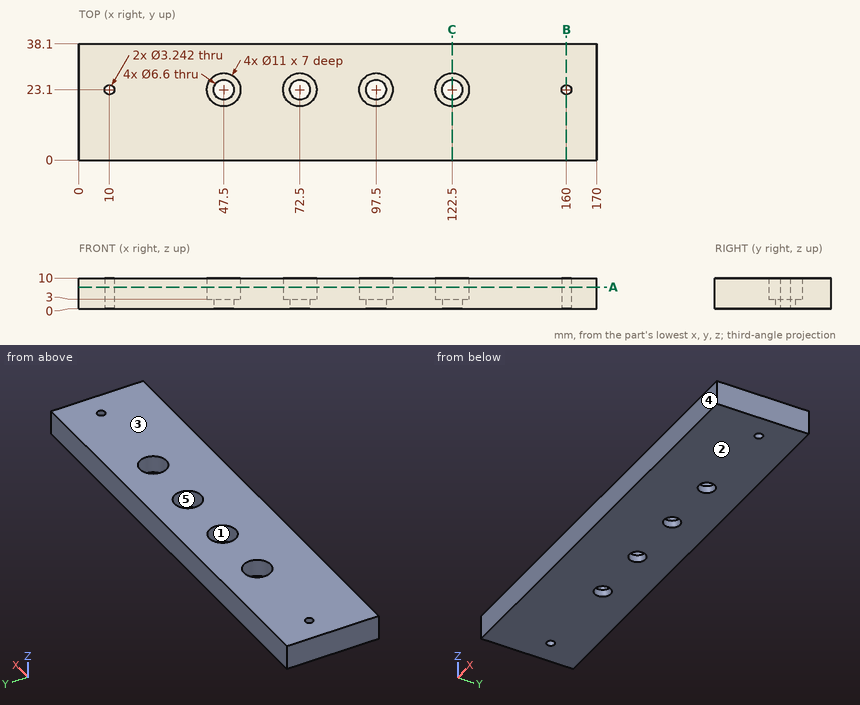
Could you check a few things on this drawing? It's one solid part, dimensions in mm from its lowest x, y, z. A direction names the side the tool comes from. Give positions to 0.01 mm unless a question says otherwise; leave off trailing zeros. Order: outer loops, then holes, each group sorted by start corner. A loop starts at its lowest first (then second) coordinate and runs counter-clockwise, first axis right, second up. Notation, with made-up numbers: (-29.75, 67.25) - (-16.75, 67.25) arc R23 ccw to (-16.75, 88.25) - close; hole circle Ø10 at (-21, 29.5). An arc over 180 degrees is marked (long way). Answer as a JSON object with one key per item and string values. Group by question number.
Item 1: If we mould it in two halves opening along Y, with no side actions, what happens to the marked faces 3, 4 and 5? For each: pulls with the +Y half, pulls with the -Y half, needs draft (parallel to the pull), parting line crosses it, or undercut.
Item 2: Please list where these lines run through material, in increasing order: probe 1 along Y at (x, z) = (122.5, 0.95); probe 2 along X at (y, z) = (25, 5.25); probe 3 along X at (y, z) = (28, 8.5).
Item 3: If we section it at C-C on x = 122.5: Please give me the cut outline in (y, z), and give its area (3 significant figures).
Item 4: For P1, Ø3.5, axis at x = 96, y = 22, coming from the +Z side; P2, Ø6, axis at x = 72.5, y = 23.1, coming from the -Z side, each with a flat end and sliding along its axis, tell me the tip position at first contact or that it passes through.
Item 5: If we section it at B-B on x = 160: Please give me the cut outline in (y, z), and give its area (3 significant figures).
Item 6: Which directions (+Z, -Z, +X, -X, +Y, -Y) give clear straight access to the entire face, cutting with the end or side of a thin tool? Please do the marked faces 1 and 2.
Item 7: If we section it at A-A on z = 7: Please give me the cut outline in (x, y), and give its area (3 significant figures).
Result set:
{
 "1": {"face 3": "needs draft", "face 4": "pulls with the -Y half", "face 5": "undercut"},
 "2": {"probe 1": "0 to 19.8, 26.4 to 38.1", "probe 2": "0 to 42.34, 52.66 to 67.34, 77.66 to 92.34, 102.66 to 117.34, 127.66 to 170", "probe 3": "0 to 45, 50 to 70, 75 to 95, 100 to 120, 125 to 170"},
 "3": {"outline": "(0, 0) - (19.8, 0) - (19.8, 3) - (17.6, 3) - (17.6, 10) - (0, 10) - close; (26.4, 0) - (38.1, 0) - (38.1, 10) - (28.6, 10) - (28.6, 3) - (26.4, 3) - close", "area": "284 mm²"},
 "4": {"P1": "z = 3", "P2": "through"},
 "5": {"outline": "(0, 0) - (21.48, 0) - (21.48, 10) - (0, 10) - close; (24.72, 0) - (38.1, 0) - (38.1, 10) - (24.72, 10) - close", "area": "349 mm²"},
 "6": {"face 1": "+Z", "face 2": "-Z, +X, -X, +Y, -Y"},
 "7": {"outline": "(0, 0) - (170, 0) - (170, 38.1) - (0, 38.1) - close; hole circle Ø3.24 at (10, 23.1); hole circle Ø11 at (47.5, 23.1); hole circle Ø11 at (72.5, 23.1); hole circle Ø11 at (97.5, 23.1); hole circle Ø11 at (122.5, 23.1); hole circle Ø3.24 at (160, 23.1)", "area": "6,080 mm²"}
}
